Source: three-view drawing plus pictorial views. Frame: mm from the lowest corner of the part. Coordinates: 2 decimals unless noted, no trailing zeros. Write each loop counter-clockwise with the first axis right and the second up, starting at its lowest first coordinate (ties: lowest second). Pieces come first, ordered by that corner, then holes. Notation, with made-up numbers: (71.25, 71.5) -> (75.25, 71.5) arc R22 cw to (75.25, 85.5) -> close; hole circle Ø1 at (67.25, 20.25). An arc over 180 degrees is marked (long way). One line per item, written item: value.
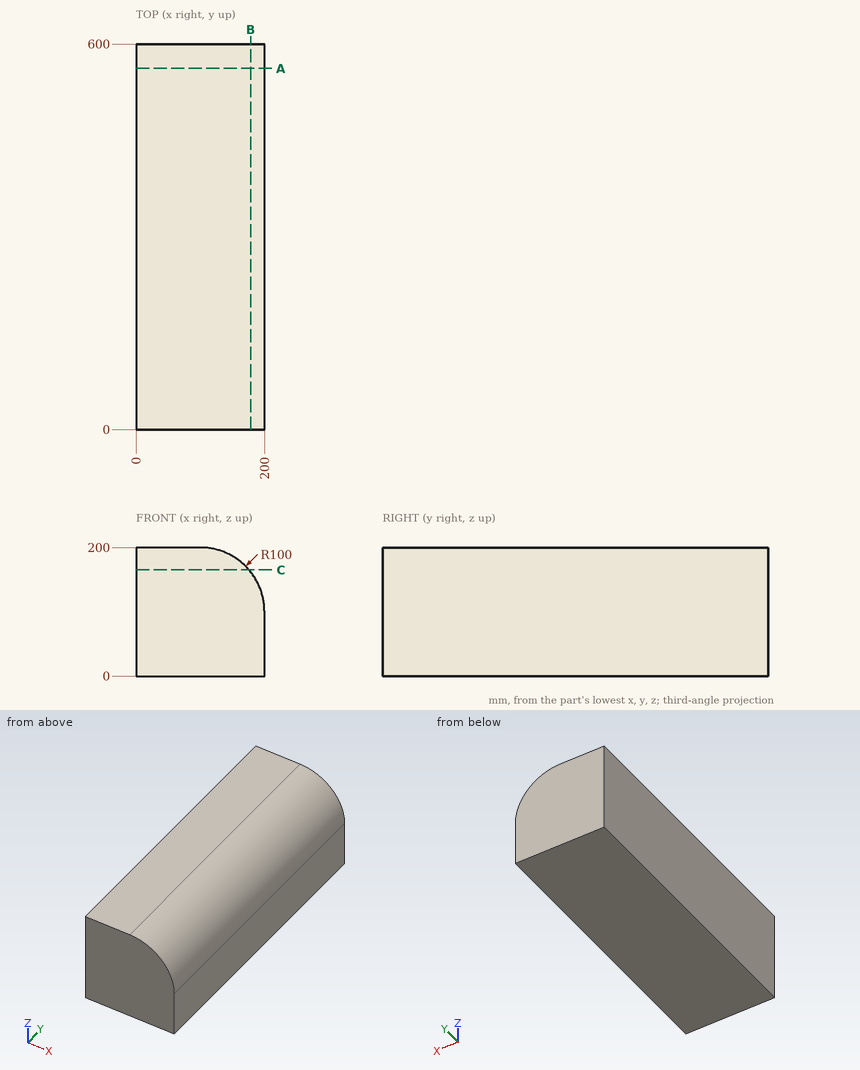
(1) Section B-B (x = 178.5). Return the cut outline in (y, z).
Responses:
outline: (0, 0) -> (600, 0) -> (600, 161.95) -> (0, 161.95) -> close
(2) Section A-A (y = 562). Return the cut outline in (x, z).
Responses:
outline: (0, 0) -> (200, 0) -> (200, 100) arc R100 ccw to (100, 200) -> (0, 200) -> close
(3) Line query: line 1 (Z direction, x = 101, y = 437.5) (3 decimals); line 2 (X direction, y = 297, z = 102.5); line 3 (Z direction, x = 186, y = 498). Output: solid intervals per line, ascending. Write a range as [from, to].
Responses:
line 1: z = [0, 199.995]
line 2: x = [0, 199.97]
line 3: z = [0, 151.03]
(4) First-contact query: pin 1 (6 mm diameter, centred on x = 77.5, y = 479.5, fed in from -Z); pin 2 (8 mm diameter, centred on x = 151.5, y = 417, fed in from +Z); pin 3 (8 mm diameter, centred on y = 69, z = 160.5, fed in from +X). Flat tips, straight axial feed; report the tip coordinate or a pass-through.
Responses:
pin 1: stops at z = 0
pin 2: stops at z = 188
pin 3: stops at x = 182.51
(5) Section C-C (z = 165). Return the cut outline in (x, y), then the cut area to 3 significant figures.
Responses:
outline: (0, 0) -> (175.99, 0) -> (175.99, 600) -> (0, 600) -> close
area: 106,000 mm2
